Geometry: see drawing. Coordinates: mm, zero at the bounding-box minimum. Coordinates: 2 decimals unless noted, no trailing zeros. Order: outer loops, then holes, each group sorted by start corner. A loop starts at its lowest first (then second) coordinate and runs counter-clockwise, first axis right, second up.
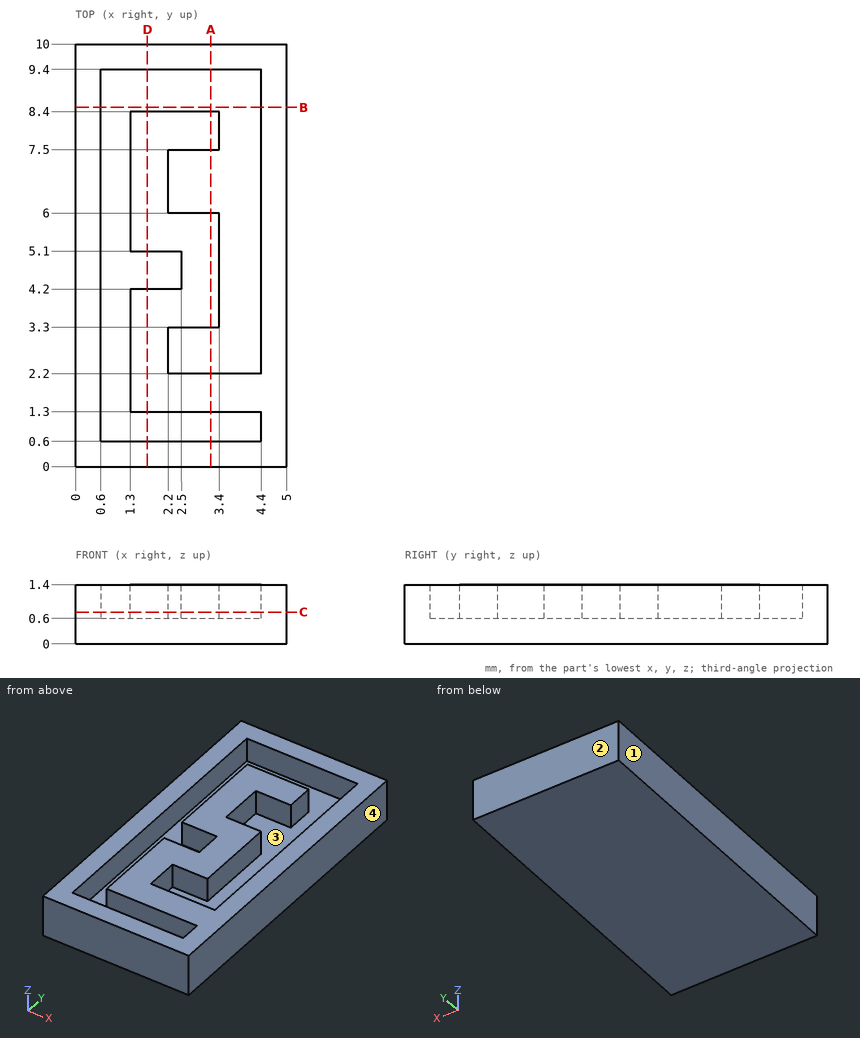
Q1. Material intervals for line 1 along Y through (x, z) = (3.8, 0.7); line 2 along Y through (x, z) = (1.75, 0.7); line 3 along Y through (x, z) = (2.6, 1.35), sorted ascending.
Solutions:
line 1: y = 0 to 0.6, 1.3 to 2.2, 9.4 to 10
line 2: y = 0 to 0.6, 1.3 to 4.2, 5.1 to 8.4, 9.4 to 10
line 3: y = 0 to 0.6, 1.3 to 2.2, 3.3 to 6, 7.5 to 8.4, 9.4 to 10
Q2. Pull-direction query (X, two-part tool) for the marked faces 1, 2, 3 and 4; classes: pulls with the +X half, pulls with the -X half, needs draft (parallel to the pull), parting line crosses it, or undercut.
Solutions:
face 1: pulls with the -X half
face 2: needs draft
face 3: undercut
face 4: pulls with the +X half
Q3. Section query D-D on x = 1.7. Output: boundary loops of the cut face in (y, z), plus the area to 3 significant figures.
Solutions:
outline: (0, 0) - (10, 0) - (10, 1.4) - (9.4, 1.4) - (9.4, 0.6) - (8.4, 0.6) - (8.4, 1.4) - (5.1, 1.4) - (5.1, 0.6) - (4.2, 0.6) - (4.2, 1.4) - (1.3, 1.4) - (1.3, 0.6) - (0.6, 0.6) - (0.6, 1.4) - (0, 1.4) - close
area: 11.9 mm2
Q4. Section query A-A on x = 3.2. Output: boundary loops of the cut face in (y, z), plus the area to 3 significant figures.
Solutions:
outline: (0, 0) - (10, 0) - (10, 1.4) - (9.4, 1.4) - (9.4, 0.6) - (8.4, 0.6) - (8.4, 1.4) - (7.5, 1.4) - (7.5, 0.6) - (6, 0.6) - (6, 1.4) - (3.3, 1.4) - (3.3, 0.6) - (2.2, 0.6) - (2.2, 1.4) - (1.3, 1.4) - (1.3, 0.6) - (0.6, 0.6) - (0.6, 1.4) - (0, 1.4) - close
area: 10.6 mm2
Q5. Section query B-B on y = 8.5. Output: boundary loops of the cut face in (x, z).
Solutions:
outline: (0, 0) - (5, 0) - (5, 1.4) - (4.4, 1.4) - (4.4, 0.6) - (0.6, 0.6) - (0.6, 1.4) - (0, 1.4) - close
Q6. Section query C-C on z = 0.75. Output: boundary loops of the cut face in (x, y).
Solutions:
outline: (0, 0) - (5, 0) - (5, 10) - (0, 10) - close; hole (0.6, 0.6) - (4.4, 0.6) - (4.4, 1.3) - (1.3, 1.3) - (1.3, 4.2) - (2.5, 4.2) - (2.5, 5.1) - (1.3, 5.1) - (1.3, 8.4) - (3.4, 8.4) - (3.4, 7.5) - (2.2, 7.5) - (2.2, 6) - (3.4, 6) - (3.4, 3.3) - (2.2, 3.3) - (2.2, 2.2) - (4.4, 2.2) - (4.4, 9.4) - (0.6, 9.4) - close
